from build123d import *

# Parameters (mm, degrees)
SKETCH052_R     = 16.6
PAD033_DEPTH    = 3
SKETCH053_W     = 4.4
SKETCH053_H     = 2.4
SKETCH053_W_2   = 2.4
SKETCH053_H_2   = 4.4
POCKET019_DEPTH = 5
PAD034_DEPTH    = 40
POCKET020_DEPTH = 31.0155254063


with BuildPart() as part:
    # Sketch052 (on Face35 of Binder010) → Pad033 (new body)
    with BuildSketch(Plane.XY.offset(6.2)):
        with Locations((-83.6396103068, 83.6396103068)):
            Circle(SKETCH052_R)
    extrude(amount=PAD033_DEPTH)

    # Sketch053 (on Face35 of Binder010) → Pocket019 (cut)
    with BuildSketch(Plane.XY.offset(6.2)):
        Polygon((-91.4177848998, 95.660425587), (-95.660425587, 91.4177848998), (-91.4177848998, 87.1751442127), (-87.1751442127, 91.4177848998), align=None)
        Polygon((-80.1040764009, 91.4177848998), (-75.8614357137, 95.660425587), (-71.6187950266, 91.4177848998), (-75.8614357137, 87.1751442127), align=None)
        Polygon((-75.8614357137, 80.1040764009), (-71.6187950266, 75.8614357137), (-75.8614357137, 71.6187950266), (-80.1040764009, 75.8614357137), align=None)
        Polygon((-87.1751442127, 75.8614357137), (-91.4177848998, 80.1040764009), (-95.660425587, 75.8614357137), (-91.4177848998, 71.6187950266), align=None)
        with Locations((-98.6396103068, 83.6396103068)):
            Rectangle(SKETCH053_W, SKETCH053_H)
        with Locations((-83.6396103068, 68.6414357137)):
            Rectangle(SKETCH053_W_2, SKETCH053_H_2)
        with Locations((-68.6414357137, 83.6396103068)):
            Rectangle(SKETCH053_W, SKETCH053_H)
        with Locations((-83.6396103068, 98.6396103068)):
            Rectangle(SKETCH053_W_2, SKETCH053_H_2)
    extrude(amount=POCKET019_DEPTH, mode=Mode.SUBTRACT)

    # Sketch054 (on Face4 of Pocket019) → Pad034 (join)
    with BuildSketch(Plane.XY.offset(9.2)):
        Polygon((-79.1848375853, 98.8424061023), (-98.8424061023, 79.1848375853), (-96.0139789776, 76.3564104606), (-76.3564104606, 96.0139789776), align=None)
        Polygon((-71.265241636, 90.922810153), (-90.922810153, 71.265241636), (-88.0943830283, 68.4368145113), (-68.4368145113, 88.0943830283), align=None)
    extrude(amount=PAD034_DEPTH)

    # Sketch055 (on Face39 of Pad034) → Pocket020 (cut, through all)
    with BuildSketch(Plane(origin=(-89.0136218438, 89.0136218438, 0), x_dir=(-0.7071067812, -0.7071067812, 0), z_dir=(-0.7071067812, 0.7071067812, 0))):
        Polygon((-3, 9.4), (3, 9.4), (3, 13.4), (0, 17.4), (-3, 13.4), align=None)
    extrude(amount=-POCKET020_DEPTH, mode=Mode.SUBTRACT)


solid = part.part
Source: CAD feature listing. Evaluate the final solid. Frame: model axes, mm. A direction names the side the tool comes from. Give positions to 0.01 mm unless a question says otherwise; leave off trailing zeros. Write each loop counter-clockwise with the first axis right and the second up, starting at its lowest first coordinate (ties: lowest second). Pieces come first, ordered by that corner, then holes. Notation, with made-up numbers: M -29,38.25 L -14,38.25 A25 ccw -14,72.25 Z; hole C -15.75,48.5 d10. An arc over 180 degrees is marked long. Answer as a JSON object with one key per item and string values.
Q1. Cut plane D-D, the plane x = -93. Return the cut outline in (y, z).
Geometry check:
{"outline": "M 69.93,6.2 L 73.2,6.2 L 73.2,9.2 L 69.93,9.2 Z; M 78.52,6.2 L 88.76,6.2 L 88.76,9.2 L 85.03,9.2 L 85.03,49.2 L 79.37,49.2 L 79.37,9.2 L 78.52,9.2 Z; M 94.08,6.2 L 97.35,6.2 L 97.35,9.2 L 94.08,9.2 Z"}
Q2. Contact query for flat-ended pins moving along their axis: P1, Ø1.2, axis at x = -84, z = 7, coming from the +Y side; P2, Ø2.5, axis at y = 98, z = 7.5, coming from the -X side; P3, Ø3, axis at x = -82, z = 30, coming from the -Y side; P4, Ø1.9, axis at y = 84, z = 7.5, coming from the -X side. Output: stop coordinate, or through.
Geometry check:
{"P1": "stops at y = 96.44", "P2": "stops at x = -93.82", "P3": "stops at y = 73.03", "P4": "stops at x = -100.2"}
Q3. Access query for faces 1 (the face through (-98, 82.44, 8)), 2 (the face through (-93.6, 73.8, 7.7)), 3 (the face through (-88.88, 89.15, 28.92)). Directions: +Z, -Z, +X, -X, +Y, -Y. A direction counts if a zero-diameter tool reaches every point of the face in a straight line with its end or side. Return the directions, or none.
Geometry check:
{"face 1": "+Z, -Z, -X", "face 2": "+Z, -Z", "face 3": "+Z, -X, +Y"}
Q4. Cut plane A-A, the plane z = 31. Return the cut outline in (x, y).
Geometry check:
{"outline": "M -98.84,79.18 L -96.01,76.36 L -76.36,96.01 L -79.18,98.84 Z; M -90.92,71.27 L -88.09,68.44 L -68.44,88.09 L -71.27,90.92 Z"}
Q5. Mould query, pull axis Z, two halves, no side actions, for faces 4 (the face through (-89.27, 93.51, 7.68)), 5 (the face through (-78.654, 80.745, 15.428)), 6 (the face through (-86.573, 88.665, 15.428)). Classes: +Z half, -Z half, draft (parallel to the pull), parting line (faces both ways), or undercut.
Geometry check:
{"face 4": "draft", "face 5": "undercut", "face 6": "undercut"}
Q6. Cut plane C-C, the plane y = 97.5. Return the cut outline in (x, z), then the cut area to 3 significant figures.
Geometry check:
{"outline": "M -92.77,6.2 L -84.84,6.2 L -84.84,9.2 L -92.77,9.2 Z; M -82.44,6.2 L -74.5,6.2 L -74.5,9.2 L -77.84,9.2 L -77.84,49.2 L -80.53,49.2 L -80.53,9.2 L -82.44,9.2 Z", "area": "155 mm^2"}
Q7. Ray query, line 1 along X through (y, z) = (87, 32); line 2 along Y through (x, z) = (-82, 37.5); line 3 along Z through (x, y) = (-98, 76.5). Return the intervals inside material, ascending.
Geometry check:
{"line 1": "x = -91.03 to -85.37, -75.19 to -69.53", "line 2": "y = 74.53 to 80.19, 90.37 to 96.03", "line 3": "z = 6.2 to 9.2"}
Q8. Cut plane B-B, the plane x = -98. Return the cut outline in (y, z).
Geometry check:
{"outline": "M 75.31,6.2 L 82.44,6.2 L 82.44,9.2 L 80.03,9.2 L 80.03,49.2 L 78.34,49.2 L 78.34,9.2 L 75.31,9.2 Z; M 84.84,6.2 L 91.97,6.2 L 91.97,9.2 L 84.84,9.2 Z"}
